Part model, mm, in its own coordinate system. Coordinates: 2 decimals unless noted, no trailing zeros. Loops run counter-clockwise (first coordinate to the right, second up) from the corner with the lowest first, then second, coordinate; pieces in that order, holes last.
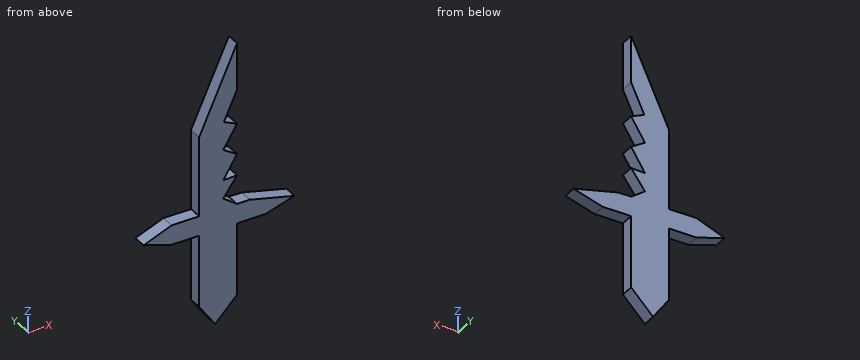
```python
from build123d import *

# Parameters (mm, degrees)
F1_DEPTH = 5.715


with BuildPart() as f1:
    # F0 (on Front) → F1 (new body)
    with BuildSketch(Plane.XZ):
        Polygon((-9.904526, 23.375541), (-9.904526, 43.280635), (-25.999382, 8.202187), (-25.999382, -25.844624), (-9.936704, -25.844624), (-15.785338, -21.608118), (-9.904526, -13.489466), (-15.785338, -13.773482), (-9.904526, -4.36581), (-15.785338, -0.689667), (-9.904526, 8.718005), (-15.493959, 11.193473), align=None)
        Polygon((-9.936704, -25.844624), (-25.999382, -25.844624), (-37.761007, -25.844624), (-49.625799, -30.48737), (-37.761007, -34.201566), (-25.999382, -34.201566), (-9.904526, -34.201566), (2.166617, -34.201566), (14.547272, -30.48737), (-4.487994, -25.844624), (-9.904526, -25.844624), (-9.904526, -25.867933), align=None)
        Polygon((-9.904526, -25.844624), (-9.936704, -25.844624), (-9.904526, -25.867933), align=None)
        Polygon((-9.904526, -34.201566), (-25.999382, -34.201566), (-25.999382, -64.843699), (-19.190019, -74.438706), (-9.904526, -64.843699), align=None)
    extrude(amount=F1_DEPTH)


solid = f1.part
```
Q1. Probe line 1 (Z direction, x = -11, y = -2.7); line 2 (X direction, y = -2.95, z = -59); line 3 (Z direction, x = -9, y = -3.35). List the from-to ranges inside material, lowest first.
Q2. Saw through at C-C (x = -31). List the corners of the cut face in (y, z) (3 decimals), plus the area to 3 significant figures.
Q3. Drop flat-ended pins along their axis: P1, Ø3, axis at x = -34, y = -2, coming from the -Z side; P2, Ø2, axis at y = -4, z = -15.5, coming from the -X side; P3, Ø1.7, axis at y = -3, z = -47, coming from the +X side. Give the stop position or say it passes through.
Q4. Saw through at B-B (z = -50). List the corners of the cut face in (x, y) (3 decimals).
Q5. Saw through at A-A (y = -4.65). List the corners of the cut face in (x, z).
Checked values:
1. line 1: z = -65.98 to -25.07, -15 to -13.54, -6.12 to -3.68, 6.97 to 9.2, 20.99 to 40.89
1. line 2: x = -26 to -9.9
1. line 3: z = -34.2 to -25.84
2. outline: (-5.715, -34.202) - (0, -34.202) - (0, -25.845) - (-5.715, -25.845) - close
2. area: 47.8 mm2
3. P1: stops at z = -34.2
3. P2: stops at x = -26
3. P3: stops at x = -9.9
4. outline: (-25.999, -5.715) - (-9.905, -5.715) - (-9.905, 0) - (-25.999, 0) - close
5. outline: (-49.63, -30.49) - (-37.76, -34.2) - (-26, -34.2) - (-26, -64.84) - (-19.19, -74.44) - (-9.9, -64.84) - (-9.9, -34.2) - (2.17, -34.2) - (14.55, -30.49) - (-4.49, -25.84) - (-9.94, -25.84) - (-15.79, -21.61) - (-9.9, -13.49) - (-15.79, -13.77) - (-9.9, -4.37) - (-15.79, -0.69) - (-9.9, 8.72) - (-15.49, 11.19) - (-9.9, 23.38) - (-9.9, 43.28) - (-26, 8.2) - (-26, -25.84) - (-37.76, -25.84) - close
